Can you work these out from the model? Positions are in its coordinate system, mm. Face numbers are marked on the shaded views. A direction names the side the tool comes from. Give positions to 0.01 mm unless a question says otherwise; leave off trailing zeros. Write each loop counter-clockwise with the first axis right and the second up, starting at its lowest first coordinate (ties: lowest second). Pieces come first, ordered by that corner, then holes. Notation, with made-up numbers: (16.5, 4.5) - (64.5, 4.5) arc R22 cw to (64.5, 27.5) - close; hole circle Ø6 at (-5, -2.75). An arc over 180 degrees is marked (long way). Use a Markdown table: item, result. Add a question column.
```python
from build123d import *

# Parameters (mm, degrees)
SM_BASE_FLANGE_2_DEPTH      = 48
SM_BASE_FLANGE_2_DEPTH_BACK = 20
SKETCH_8_R                  = 11
SKETCH_8_R_2                = 1.5
CUT_EXTRUDE_1_DEPTH         = 66.984846745
SKETCH_10_R                 = 14
SKETCH_10_R_2               = 2
EXTRUDE_1_DEPTH             = 4
SKETCH_11_R                 = 2
CUT_EXTRUDE_2_DEPTH         = 99.371743911
FILLET_1_R                  = 5
SKETCH_13_R                 = 3
CUT_EXTRUDE_3_DEPTH         = 99.371743911


# Sheet-metal steps are written as plain solids
with BuildPart() as part:
    # Sketch 1 → 基体-法兰2 (new, two sides: drawn at the far end of the back side and taken through both)
    with BuildSketch(Plane.XY.offset(-SM_BASE_FLANGE_2_DEPTH_BACK)):
        with BuildLine():
            Line((-33, 35), (-33, 6))
            ThreePointArc((-33, 6), (-31.242640687, 1.757359313), (-27, 0))
            Line((-27, 0), (27, 0))
            ThreePointArc((27, 0), (31.242640687, 1.757359313), (33, 6))
            Line((33, 6), (33, 35))
            Line((33, 35), (29, 35))
            Line((29, 35), (29, 6))
            ThreePointArc((29, 6), (28.414213562, 4.585786438), (27, 4))
            Line((27, 4), (-27, 4))
            ThreePointArc((-27, 4), (-28.414213562, 4.585786438), (-29, 6))
            Line((-29, 6), (-29, 35))
            Line((-29, 35), (-33, 35))
        make_face()
    extrude(amount=SM_BASE_FLANGE_2_DEPTH + SM_BASE_FLANGE_2_DEPTH_BACK)

    # 草图8 → 切除-拉伸1 (cut, through all)
    with BuildSketch(Plane(origin=(0, 4, 0), x_dir=(1, 0, 0), z_dir=(0, 1, 0))):
        with Locations(Location((0, -24, 0), (0, 0, 270))):
            Circle(SKETCH_8_R)
        with Locations(Location((0, -10, 0), (0, 0, 270))):
            Circle(SKETCH_8_R_2)
        with Locations(Location((14, -24, 0), (0, 0, 270))):
            Circle(SKETCH_8_R_2)
        with Locations(Location((0, -38, 0), (0, 0, 270))):
            Circle(SKETCH_8_R_2)
        with Locations(Location((-14, -24, 0), (0, 0, 270))):
            Circle(SKETCH_8_R_2)
    extrude(amount=-CUT_EXTRUDE_1_DEPTH, mode=Mode.SUBTRACT)

    # 草图10 → 凸台-拉伸1 (add)
    with BuildSketch(Plane(origin=(0, 4, 0), x_dir=(1, 0, 0), z_dir=(0, 1, 0))):
        with BuildLine():
            Line((-23, 41), (-23, 20))
            Line((-23, 20), (23, 20))
            Line((23, 20), (23, 41))
            ThreePointArc((23, 41), (0, 64), (-23, 41))
        make_face()
        with Locations(Location((0, 41, 0), (0, 0, 270))):
            Circle(SKETCH_10_R, mode=Mode.SUBTRACT)
        with Locations(Location((0, 58.5, 0), (0, 0, 270))):
            Circle(SKETCH_10_R_2, mode=Mode.SUBTRACT)
        with Locations(Location((17.5, 41, 0), (0, 0, 270))):
            Circle(SKETCH_10_R_2, mode=Mode.SUBTRACT)
        with Locations(Location((0, 23.5, 0), (0, 0, 270))):
            Circle(SKETCH_10_R_2, mode=Mode.SUBTRACT)
        with Locations(Location((-17.5, 41, 0), (0, 0, 270))):
            Circle(SKETCH_10_R_2, mode=Mode.SUBTRACT)
    extrude(amount=-EXTRUDE_1_DEPTH)

    # 草图11 → 切除-拉伸2 (cut, through all)
    with BuildSketch(Plane.ZY.offset(33)):
        with Locations((19, 18)):
            Circle(SKETCH_11_R)
        with Locations((9, 18)):
            Circle(SKETCH_11_R)
        with Locations(Location((29, 18, 0), (0, 0, 180))):
            Circle(SKETCH_11_R)
        with Locations(Location((39, 18, 0), (0, 0, 180))):
            Circle(SKETCH_11_R)
        with Locations((19, 28)):
            Circle(SKETCH_11_R)
        with Locations(Location((29, 28, 0), (0, 0, 180))):
            Circle(SKETCH_11_R)
    extrude(amount=-CUT_EXTRUDE_2_DEPTH, mode=Mode.SUBTRACT)

    # 圆角1
    fillet_1_edges = [part.edges().sort_by_distance(p)[0] for p in [
        (-31, 35, -20),
        (31, 35, -20),
        (-31, 35, 48),
        (31, 35, 48),
    ]]
    fillet(fillet_1_edges, radius=FILLET_1_R)

    # 草图13 → 切除-拉伸3 (cut, through all)
    with BuildSketch(Plane(origin=(33, 0, 0), x_dir=(0, 0, -1), z_dir=(1, 0, 0))):
        with Locations((10, 28)):
            Circle(SKETCH_13_R)
        with Locations((10, 18)):
            Circle(SKETCH_13_R)
    extrude(amount=-CUT_EXTRUDE_3_DEPTH, mode=Mode.SUBTRACT)


solid = part.part
```
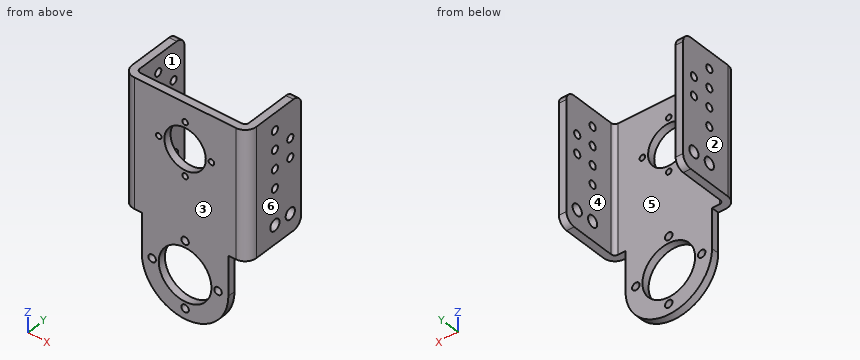
Q1. Suppose I cut it at A-A (x = 0). Please give me the cut outline in (y, z).
Q2. If I drill on probe 1 along X at (y, z) = (30.5, 20.5); probe 2 along Y at (x, z) = (31, -10); probe 3 along Y at (x, z) = (-30, 19), over which ranges is the centre line in solid material (lowest first)? Write a range as [from, to].
Q3. Suppose I cut it at D-D (y = 28). Give the number of separate pieces and of enclosed holes in the cut face, and give its area (3 significant figures).
Q4. I'm going to push flat-ended pins straight in: P1, Ø3, axis at y = 2.5, z = -35.5, coming from the -X side; P2, Ø2.5, axis at y = 18, z = 39, coming from the +X side; P3, Ø6, axis at x = 3, z = 5, coming from the +Y side; P4, Ø3, axis at y = 2, z = -35.5, coming from the +X side. Where does each tip first touch, or does it pass through?
Q5. Suppose I cut it at B-B (y = 13). Please give me the cut outline in (x, z), and give its area (3 significant figures).
Q6. Suppose I cut it at C-C (z = -23.5). Please give me the cut outline in (x, y), and give its area (3 significant figures).
Q7. On a 3-axis mill with a long thin cutter (end or side, diameter ignored), from which of +Z, -Z, +X, -X, +Y, -Y can I reach the whole of each face in a straight line? I mean the marked faces 5 and 6. Say none if no direction works.
Q8. If we mould it in two halves opening along X, with no side actions, what happens to the marked faces 1, 2, 3 and 4? For each: released by +X, released by -X, zero draft, split by the parting line, or undercut.
Derived:
| question | item | result |
|---|---|---|
| 1 | outline | (0, -64) - (4, -64) - (4, -60.5) - (0, -60.5) - close; (0, -56.5) - (4, -56.5) - (4, -55) - (0, -55) - close; (0, -27) - (4, -27) - (4, -25.5) - (0, -25.5) - close; (0, -21.5) - (4, -21.5) - (4, 8.5) - (0, 8.5) - close; (0, 11.5) - (4, 11.5) - (4, 13) - (0, 13) - close; (0, 35) - (4, 35) - (4, 36.5) - (0, 36.5) - close; (0, 39.5) - (4, 39.5) - (4, 48) - (0, 48) - close |
| 2 | probe 1 | [-33, -29], [29, 33] |
| 2 | probe 2 | [1.53, 15], [21, 25], [31, 35] |
| 2 | probe 3 | [0.8, 16], [20, 26], [30, 35] |
| 3 | separate pieces | 8 |
| 3 | enclosed holes | 0 |
| 3 | area | 432 mm² |
| 4 | P1 | x = -23 |
| 4 | P2 | through |
| 4 | P3 | y = 4 |
| 4 | P4 | x = 23 |
| 5 | outline | (-33, -20) - (-29, -20) - (-29, 48) - (-33, 48) - close; (29, -20) - (33, -20) - (33, 48) - (29, 48) - close |
| 5 | area | 544 mm² |
| 6 | outline | (-23, 0) - (-2, 0) - (-2, 4) - (-23, 4) - close; (2, 0) - (23, 0) - (23, 4) - (2, 4) - close |
| 6 | area | 168 mm² |
| 7 | face 5 | +Z, -Z, +Y |
| 7 | face 6 | +Z, -Z, +X, +Y, -Y |
| 8 | face 1 | undercut |
| 8 | face 2 | released by -X |
| 8 | face 3 | zero draft |
| 8 | face 4 | undercut |
